```python
from build123d import *

# Parameters (mm, degrees)
EXTRUDE_1_DEPTH              = 96
HOLE_WIZARD_M3_1_D           = 3.6
HOLE_WIZARD_M3_1_DEPTH       = 5
HOLE_WIZARD_M3_1_CBORE_D     = 7
HOLE_WIZARD_M3_1_CBORE_DEPTH = 2


with BuildPart() as part:
    # 草图1 → 凸台-拉伸1 (new body)
    with BuildSketch(Plane(origin=(0, 96, 0), x_dir=(1, 0, 0), z_dir=(0, 1, 0))):
        with BuildLine():
            Line((1055, -2.499371855), (1055, 2.25))
            Line((1055, 2.25), (1045, 2.25))
            Line((1045, 2.25), (1045, -2.499371855))
            ThreePointArc((1045, -2.499371855), (1050, -2.75), (1055, -2.499371855))
        make_face()
    extrude(amount=-EXTRUDE_1_DEPTH)

    # M3 六角头机械螺钉的柱形沉头孔1
    with Locations(Plane(origin=(1050, 84.5, 2.75), x_dir=(0, 1, 0), z_dir=(0, 0, 1))):
        with Locations((0, 0)):
            hole_wizard_m3_1 = CounterBoreHole(HOLE_WIZARD_M3_1_D / 2, HOLE_WIZARD_M3_1_CBORE_D / 2, HOLE_WIZARD_M3_1_CBORE_DEPTH, depth=HOLE_WIZARD_M3_1_DEPTH)

    # 镜向1: M3 六角头机械螺钉的柱形沉头孔1 across plane
    add(hole_wizard_m3_1.mirror(Plane(origin=(0, 48, 0), x_dir=(0, 0, 1), z_dir=(0, -1, 0))), mode=Mode.SUBTRACT)


solid = part.part
```
The model under review builds one solid part; all positions refer to its coordinate system, in mm. A direction names the side the tool comes from. Round coordinates to 2 decimals unless told otherwise and drop trailing zeros. Write each loop counter-clockwise with the first axis right and the second up, starting at its lowest first coordinate (ties: lowest second). Pieces come first, ordered by that corner, then holes. Notation, with made-up numbers: (88, 78.5) -> (126, 78.5) arc R29 cw to (126, 117.5) -> close; hole circle Ø8 at (6.5, 51). An arc over 180 degrees is marked (long way). Use CSV: the item, a comma, the result in double quotes.
Q1. For faces 1 (the flat face through (1048, 84, 0.75)), 2 (the cylindrical face through (1049.93, 48.67, 2.75)), list the 3-axis set-ups (+Z, -Z, +X, -X, +Y, -Y) from which the entire face can be reached by the end or side of a thin tool; tool diameter is ignored.
Checks:
face 1,"+Z"
face 2,"+Z, +Y, -Y"
Q2. Consider section D-D (y = 11.5). Give the boundary of the cut face in (x, z), then the cut area to 3 significant figures.
Checks:
outline,"(1045, -2.25) -> (1048.2, -2.25) -> (1048.2, 0.75) -> (1046.5, 0.75) -> (1046.5, 2.63) arc R50 ccw to (1045, 2.5) -> close; (1051.8, -2.25) -> (1055, -2.25) -> (1055, 2.5) arc R50 ccw to (1053.5, 2.63) -> (1053.5, 0.75) -> (1051.8, 0.75) -> close"
area,"24.7 mm²"
Q3. Consider section B-B (y = 85.5). Give the boundary of the cut face in (x, z), then the cut area to 3 significant figures.
Checks:
outline,"(1045, -2.25) -> (1048.5, -2.25) -> (1048.5, 0.75) -> (1046.65, 0.75) -> (1046.65, 2.64) arc R50 ccw to (1045, 2.5) -> close; (1051.5, -2.25) -> (1055, -2.25) -> (1055, 2.5) arc R50 ccw to (1053.35, 2.64) -> (1053.35, 0.75) -> (1051.5, 0.75) -> close"
area,"27.0 mm²"
Q4. For pin 1 Ø3.5 at (x, y) = (1050.5, 84) entering from +Z; pin 2 Ø1.5 at (x, y) = (1046.5, 73) entering from +Z; pin 3 Ø3 at (x, y) = (1050, 84.5) entering from +Z, all flat-tipped, find the tip position at first contact; note any pin that passes through.
Checks:
pin 1,"z = 0.75"
pin 2,"z = 2.67"
pin 3,"through"
Q5. Consider section A-A (x = 1050). Give the boundary of the cut face in (y, z).
Checks:
outline,"(0, -2.25) -> (9.7, -2.25) -> (9.7, 0.75) -> (8, 0.75) -> (8, 2.75) -> (0, 2.75) -> close; (13.3, -2.25) -> (82.7, -2.25) -> (82.7, 0.75) -> (81, 0.75) -> (81, 2.75) -> (15, 2.75) -> (15, 0.75) -> (13.3, 0.75) -> close; (86.3, -2.25) -> (96, -2.25) -> (96, 2.75) -> (88, 2.75) -> (88, 0.75) -> (86.3, 0.75) -> close"
Q6. To check wall thickness, follow probe 1 along Y at (x, z) = (1050, 1.6); probe 2 along Y at (x, z) = (1050, -1.4); probe 3 along X at (y, z) = (84.5, -1.5). State the ranges of each line that lie inside material, in increasing order. Write a range as [from, to].
Checks:
probe 1,"[0, 8], [15, 81], [88, 96]"
probe 2,"[0, 9.7], [13.3, 82.7], [86.3, 96]"
probe 3,"[1045, 1048.2], [1051.8, 1055]"
Q7. Consider section C-C (z = -1). Give the boundary of the cut face in (x, y).
Checks:
outline,"(1045, 0) -> (1055, 0) -> (1055, 96) -> (1045, 96) -> close; hole circle Ø3.6 at (1050, 11.5); hole circle Ø3.6 at (1050, 84.5)"
